Drawing for the job (mm, zero at the part's lowest x, y, z). A direction names the side the tool comes from. Coordinates: 2 decimals unless noted, no trailing zeros. Loops run counter-clockwise (first coordinate to the right, second up) from the corner with the lowest first, then second, coordinate; pieces in that order, holes last. Notation, with made-up numbers: (34.5, 55) - (73.5, 55) arc R14 ccw to (73.5, 82) - close; hole circle Ø5 at (-34, 69). An arc over 180 degrees is marked (long way). One line per item, written item: value.
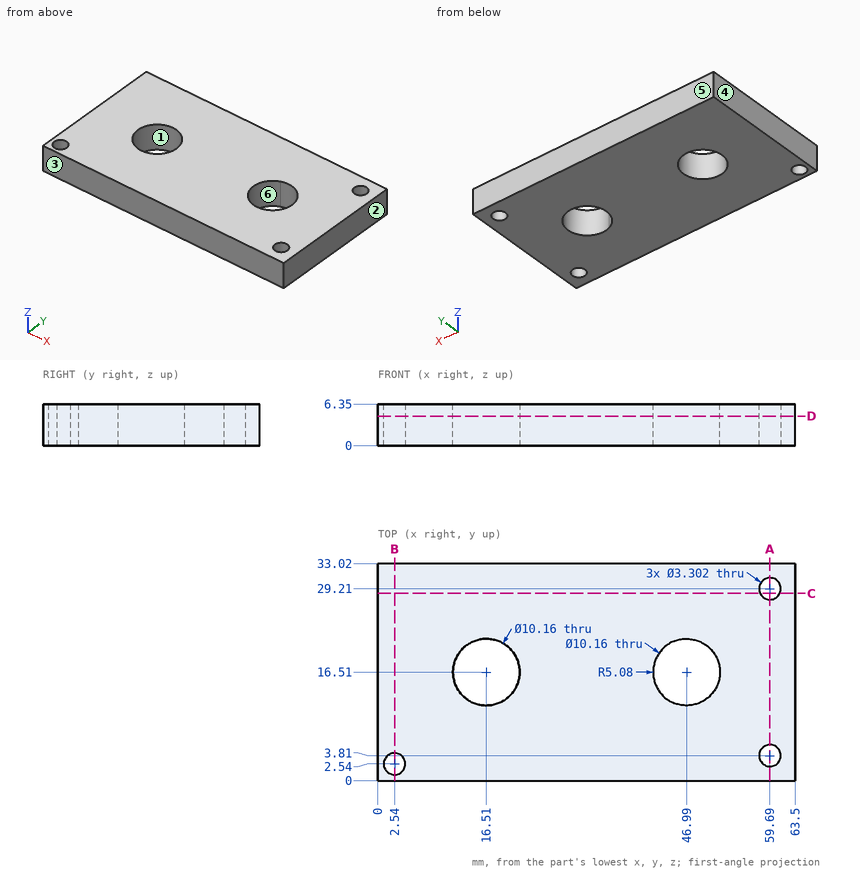
Item 1: Cut at D-D, the plane z = 4.5. Write the cut outline in (x, y) (3 decimals).
Check result:
outline: (0, 0) - (63.5, 0) - (63.5, 33.02) - (0, 33.02) - close; hole circle Ø3.302 at (2.54, 2.54); hole circle Ø10.16 at (16.51, 16.51); hole (45.085, 11.801) arc R5.08 ccw (long way) to (45.085, 21.219) arc R5.08 ccw to start; hole circle Ø3.302 at (59.69, 3.81); hole circle Ø3.302 at (59.69, 29.21)
Item 2: Cut at B-B, the plane x = 2.54. Write the cut outline in (y, z).
Check result:
outline: (0, 0) - (0.89, 0) - (0.89, 6.35) - (0, 6.35) - close; (4.19, 0) - (33.02, 0) - (33.02, 6.35) - (4.19, 6.35) - close
Item 3: Tool access for the marked faces 5 and 6: list every direction of +Z, -Z, +X, -X, +Y, -Y with a clear straight run to the whole face (end or side of a thin tool).
Check result:
face 5: +Z, -Z, +X, -X, +Y
face 6: +Z, -Z
Item 4: Probe probe 1 along X at (y, z) = (16.51, 2.5); probe 2 along Y at (x, z) = (2.54, 3.5); probe 3 along Y at (x, z) = (46.99, 5). List the from-to ranges inside material, lowest first. Write a range as from..to.
Check result:
probe 1: x = 0..11.43, 21.59..41.91, 52.07..63.5
probe 2: y = 0..0.89, 4.19..33.02
probe 3: y = 0..11.43, 21.59..33.02
Item 5: Drop flat-ended pins along their axis: P1, Ø11.5, axis at x = 16.51, y = 16.51, coming from the +Z side; P2, Ø2, axis at x = 2.54, y = 2.54, coming from the +Z side. Give the stop position or say it passes through.
Check result:
P1: stops at z = 6.35
P2: passes through
Item 6: Pull direction X, two halves, no side cores. Call the marked faces 1, 2, 3 and 4: released by +X, released by -X, zero draft, split by the parting line, or undercut.
Check result:
face 1: undercut
face 2: released by +X
face 3: zero draft
face 4: released by -X
Item 7: Cut at A-A, the plane x = 59.69. Write the cut outline in (y, z), then the cut area to 3 significant figures.
Check result:
outline: (0, 0) - (2.16, 0) - (2.16, 6.35) - (0, 6.35) - close; (5.46, 0) - (27.56, 0) - (27.56, 6.35) - (5.46, 6.35) - close; (30.86, 0) - (33.02, 0) - (33.02, 6.35) - (30.86, 6.35) - close
area: 168 mm^2
Item 8: Cut at C-C, the plane y = 28.5. Write the cut outline in (x, z).
Check result:
outline: (0, 0) - (58.2, 0) - (58.2, 6.35) - (0, 6.35) - close; (61.18, 0) - (63.5, 0) - (63.5, 6.35) - (61.18, 6.35) - close
